Verification items for the finished model (mm, model axes). Face numbers are marked on the shaded views. A direction names the side the tool comes from. Coordinates: 2 decimals unless noted, no trailing zeros. Order: outer loops, then holes, each group sorted by start corner. A loop starts at its lowest first (then second) coordinate and runs counter-clockwise, first axis right, second up. Notation, with made-up numbers: (71.25, 87.5) -> (127.25, 87.5) arc R37 cw to (127.25, 124.5) -> close; hole circle Ø6 at (79.5, -2). An arc over 180 degrees is marked (long way). Use CSV: the item, a comma, the result in double quotes. Start each with the question number.
1) Release check for a two-part mould opening along Z. For the marked faces 5, 6, 7 and 8 record: released by +Z, released by -Z, zero draft, split by the parting line, or undercut.
2) Go/stop test with flat-tipped pins: pin 1 (8 mm diameter, centred on x = 16, z = 15.5, fed in from -Y); pin 2 (0.8 mm diameter, centred on x = 4, y = -24.5, fed in from -Z) (3 decimals); pin 3 (1.1 mm diameter, centred on x = 4, y = -24.5, fed in from +Z) (3 decimals). Record where each tip stops, or that it passes through.
3) Sectioned sample at D-D on x = 11.75. Record the boundary of the cut face in (y, z) (3 decimals).
4) Sectioned sample at C-C on y = -4.5. Record the boundary of the cut face in (x, z) (3 decimals).
5) Scan lines: line 1 along Z through (x, y) = (14.5, -6.25); line 2 along X through (y, z) = (-1.75, 5); line 3 along Y through (x, z) = (2.5, 6.25). Record each from-to range of solid material in increasing order.
6) Sectioned sample at B-B on z = 4.5. Record the boundary of the cut face in (x, y), then the cut area to 3 significant figures.
7) Sectioned sample at A-A on x = 5. Record the boundary of the cut face in (y, z) (3 decimals), then the cut area to 3 significant figures.
8) Tool access check on the marked faces 1, 2, 3 and 4. Record the directions out of +Z, -Z, +X, -X, +Y, -Y that give a thin tool (end or side, any length) a straight path to the whole face; none if there is none.
from build123d import *

# Parameters (mm, degrees)
F0_W     = 20
F0_H     = 17.45
F1_DEPTH = 8
F0_W_2   = 6
F0_H_2   = 6
F0_R     = 1
F2_DEPTH = 1
F3_DEPTH = 25
F4_W     = 6
F4_H     = 6
F5_DEPTH = 1
F6_R     = 1.5
F7_W     = 5
F7_H     = 5
F8_DEPTH = 0.2
F9_R     = 1


with BuildPart() as f1:
    # F0 (on Front) → F1 (new body)
    with BuildSketch(Plane.XZ):
        with Locations((10, 8.725)):
            Rectangle(F0_W, F0_H)
        Polygon((19, 16.45), (19, 11.225), (19, 6.225), (19, 1), (1, 1), (1, 16.45), align=None, mode=Mode.SUBTRACT)
    extrude(amount=F1_DEPTH)

    # F0 (on Front) → F2 (join)
    with BuildSketch(Plane.XZ):
        Polygon((19, 11.225), (14, 11.225), (14, 15.225), (2, 15.225), (2, 11.725), (8, 11.725), (8, 5.725), (2, 5.725), (2, 2.225), (14, 2.225), (14, 6.225), (19, 6.225), align=None)
        with Locations((5, 8.725)):
            Rectangle(F0_W_2, F0_H_2)
        with Locations((5, 8.725)):
            Circle(F0_R, mode=Mode.SUBTRACT)
    extrude(amount=F2_DEPTH)

    # F0 (on Front) → F3 (join)
    with BuildSketch(Plane.XZ):
        with Locations((5, 8.725)):
            Circle(F0_R)
    extrude(amount=F3_DEPTH)

    # F4 (on face) → F5 (join)
    with BuildSketch(Plane.XZ.offset(25)):
        with Locations((5, 8.725)):
            Rectangle(F4_W, F4_H)
    extrude(amount=-F5_DEPTH)

    # F6
    f6_edges = [f1.edges().sort_by_distance(p)[0] for p in [
        (4, -24, 8.725),
        (4, -1, 8.725),
    ]]
    fillet(f6_edges, radius=F6_R)

    # F7 (on face) → F8 (cut)
    with BuildSketch(Plane.XZ.offset(1)):
        with Locations((16.5, 8.725)):
            Rectangle(F7_W, F7_H)
    extrude(amount=-F8_DEPTH, mode=Mode.SUBTRACT)

    # F9
    f9_edges = [f1.edges().sort_by_distance(p)[0] for p in [
        (2, -0.5, 15.225),
        (14, -0.5, 15.225),
        (2, -0.5, 2.225),
        (14, -0.5, 2.225),
    ]]
    fillet(f9_edges, radius=F9_R)


solid = f1.part
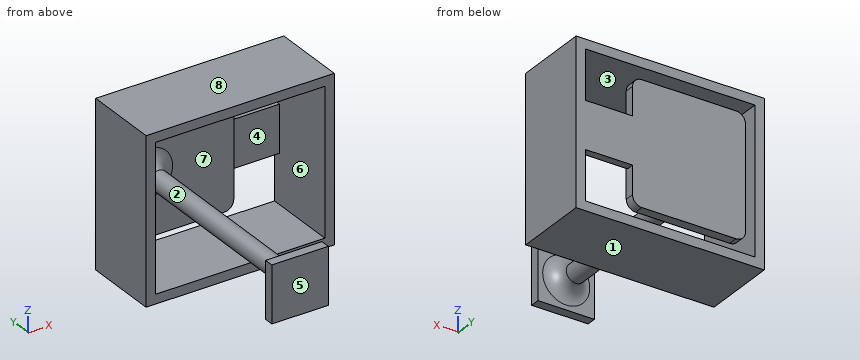
Answers follow:
1,face 5,"zero draft"
1,face 6,"undercut"
1,face 7,"undercut"
1,face 8,"released by +Z"
2,pin 1,"stops at y = -8"
2,pin 2,"stops at z = 5.725"
2,pin 3,"stops at z = 11.725"
3,outline,"(-8, 0) -> (0, 0) -> (0, 1) -> (-8, 1) -> close; (-8, 16.45) -> (0, 16.45) -> (0, 17.45) -> (-8, 17.45) -> close; (-1, 2.225) -> (0, 2.225) -> (0, 15.225) -> (-1, 15.225) -> close"
4,outline,"(0, 0) -> (20, 0) -> (20, 17.45) -> (0, 17.45) -> close; circle Ø2 at (5, 8.725); hole (1, 1) -> (19, 1) -> (19, 16.45) -> (1, 16.45) -> close"
5,line 1,"z = 0 to 1, 16.45 to 17.45"
5,line 2,"x = 0 to 1, 19 to 20"
5,line 3,"y = -25 to -24, -1 to 0"
6,outline,"(0, -8) -> (1, -8) -> (1, 0) -> (0, 0) -> close; (2, -1) -> (14, -1) -> (14, 0) -> (2, 0) -> close; (19, -8) -> (20, -8) -> (20, 0) -> (19, 0) -> close"
6,area,"28.0 mm²"
7,outline,"(-25, 5.725) -> (-24, 5.725) -> (-24, 6.225) arc R1.5 cw to (-22.5, 7.725) -> (-2.5, 7.725) arc R1.5 cw to (-1, 6.225) -> (-1, 2.225) -> (0, 2.225) -> (0, 15.225) -> (-1, 15.225) -> (-1, 11.225) arc R1.5 cw to (-2.5, 9.725) -> (-22.5, 9.725) arc R1.5 cw to (-24, 11.225) -> (-24, 11.725) -> (-25, 11.725) -> close; (-8, 0) -> (0, 0) -> (0, 1) -> (-8, 1) -> close; (-8, 16.45) -> (0, 16.45) -> (0, 17.45) -> (-8, 17.45) -> close"
7,area,"82.9 mm²"
8,face 1,"-Z, +X, -X, +Y, -Y"
8,face 2,"none"
8,face 3,"+Y, -Y"
8,face 4,"-Y"
